Build history of the part. All positions in model axes, mm. Round coordinates to 2 decimals unless told otherwise and drop trailing zeros. Write each loop counter-clockwise with the first axis right and the second up, starting at its lowest first coordinate (ties: lowest second). Pieces come first, ordered by that corner, then holes. Notation, with made-up numbers: M -40,54 L 14,54 A9 ccw 14,70 Z; hole C 23,74 d6. An arc over 180 degrees is marked long. Use a Markdown table: item, result.
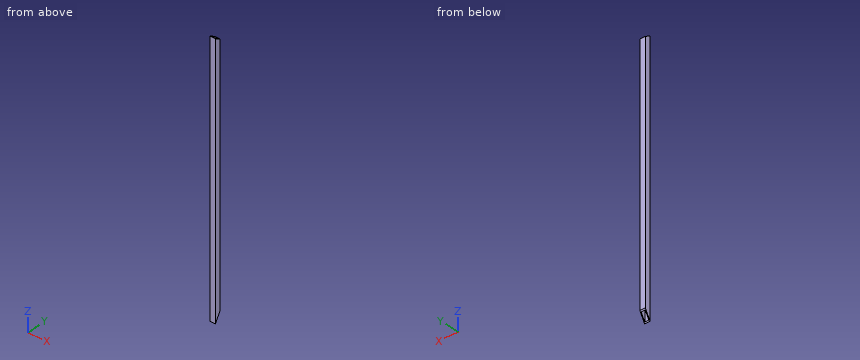
Autodesk Inventor part; units mm, degrees
ref_plane "YZ Plane" through (0, 0, 0) normal (1, 0, 0) x (0, 1, 0)
ref_plane "XZ Plane" through (0, 0, 0) normal (0, 1, 0) x (-1, 0, 0)
ref_plane "XY Plane" through (0, 0, 0) normal (0, 0, 1) x (1, 0, 0)
sketch "Sketch1" plane through (0, 0, 0) normal (0, 0, 1) x (1, 0, 0)
  line L0 (-12.7, -12.7) -> (12.7, -12.7)
  line L1 (12.7, -12.7) -> (12.7, 12.7)
  line L2 (12.7, 12.7) -> (-12.7, 12.7)
  line L3 (-12.7, 12.7) -> (-12.7, -12.7)
  line L4 (-12.7, -12.7) -> (12.7, 12.7) construction
  line L5 (12.7, -12.7) -> (-12.7, 12.7) construction
  line L6 (-9.525, -9.525) -> (9.525, -9.525)
  line L7 (9.525, -9.525) -> (9.525, 9.525)
  line L8 (9.525, 9.525) -> (-9.525, 9.525)
  line L9 (-9.525, 9.525) -> (-9.525, -9.525)
  line L10 (-9.525, -9.525) -> (9.525, 9.525) construction
  line L11 (9.525, -9.525) -> (-9.525, 9.525) construction
  point P0 (0, 0)
  dimension "d0" = 25.4
  dimension "d1" = 3.175
extrude "Extrusion1" add sketch "Sketch1" along normal mid plane 1219.2
sketch "Sketch3" plane through (12.7, -12.7, 609.6) normal (1, 0, 0) x (0, 0, -1)
  line L0 (1219.2, 25.4) -> (0, 25.4)
  line L1 (0, 0) -> (1219.2, 0)
  line L2 (0, 25.4) -> (0, 0)
  line L3 (0, 0) -> (14.6647, 25.4)
  line L4 (1219.2, 0) -> (1219.2, 25.4)
  line L5 (1219.2, 22.225) -> (1219.2, 3.175)
  line L6 (1175.2059, 25.4) -> (1219.2, 0)
  point P0 (609.6, 12.7)
  dimension "d6" = 30
  dimension "d7" = 60
extrude "Extrusion3" cut sketch "Sketch3" against normal through all contours L4 L6 L0 | L3 L2 L0
properties part number "30-60-supportBrace"
Q1. Cut at C-C on y = 2. Give the cut face in (x, z) (3 decimals).
Response values:
| item | result |
|---|---|
| outline | M -12.7,-584.139 L -9.525,-584.139 L -9.525,601.113 L -12.7,601.113 Z; M 9.525,-584.139 L 12.7,-584.139 L 12.7,601.113 L 9.525,601.113 Z |
Q2. Cut at A-A on x = -1.5. Give the cut face in (y, z) (3 decimals).
Response values:
| item | result |
|---|---|
| outline | M -12.7,-609.6 L -9.525,-604.101 L -9.525,607.767 L -12.7,609.6 Z; M 9.525,-571.105 L 12.7,-565.606 L 12.7,594.935 L 9.525,596.768 Z |
Q3. Drill centre lines: L1, parallel to Y at x = -4, z = 357.5 (3 decimals); L2, parallel to Z at x = 11.75, y = 0.25. Where is each one in solid material? Low to high.
Response values:
| item | result |
|---|---|
| L1 | y = -12.7 to -9.525, 9.525 to 12.7 |
| L2 | z = -587.17 to 602.12 |
Q4. Cut at B-B on z = -496.5. Give the cut face in (x, y) (3 decimals).
Response values:
| item | result |
|---|---|
| outline | M -12.7,-12.7 L 12.7,-12.7 L 12.7,12.7 L -12.7,12.7 Z; hole M -9.525,-9.525 L 9.525,-9.525 L 9.525,9.525 L -9.525,9.525 Z |
Q5. Drop a flat-ended pin along its axis: P1, Ø10, axis at x = -8.5, y = -5, coming from the -Z side. Give the stop position or say it passes through.
Response values:
| item | result |
|---|---|
| P1 | stops at z = -604.92 |
